```python
from build123d import *

# Parameters (mm, degrees)
ESQUISSE1_R        = 1.5
BOSS_EXTRU_2_DEPTH = 3


with BuildPart() as part:
    # Esquisse1 → Boss.-Extru.2 (new body)
    with BuildSketch(Plane.XY):
        with BuildLine():
            Line((10, -16.155494421), (10, -33.155494421))
            Line((10, -33.155494421), (-10, -33.155494421))
            Line((-10, -33.155494421), (-10, -16.155494421))
            ThreePointArc((-10, -16.155494421), (0, 19), (10, -16.155494421))
        make_face()
        with Locations((0, 14)):
            Circle(ESQUISSE1_R, mode=Mode.SUBTRACT)
        with Locations((12.124355653, -7)):
            Circle(ESQUISSE1_R, mode=Mode.SUBTRACT)
        with Locations((-12.124355653, -7)):
            Circle(ESQUISSE1_R, mode=Mode.SUBTRACT)
        with BuildLine():
            ThreePointArc((-2.411034891, 11.820685714), (0, 10.75), (2.411034891, 11.820685714))
            ThreePointArc((2.411034891, 11.820685714), (3.975330286, 12.779130538), (5.80943088, 12.737759334))
            ThreePointArc((5.80943088, 12.737759334), (11.865562564, 7.430237213), (13.995977593, -0.335575935))
            ThreePointArc((13.995977593, -0.335575935), (13.382779595, -2.564868949), (11.442531564, -3.822325392))
            ThreePointArc((11.442531564, -3.822325392), (9.309773091, -5.375), (9.031496673, -7.998360322))
            ThreePointArc((9.031496673, -7.998360322), (9.079386541, -9.832302285), (8.126507731, -11.399994391))
            ThreePointArc((8.126507731, -11.399994391), (0.5019929, -13.990997217), (-7.288606081, -11.953084179))
            ThreePointArc((-7.288606081, -11.953084179), (-8.912631465, -10.307392628), (-9.031496673, -7.998360322))
            ThreePointArc((-9.031496673, -7.998360322), (-9.309773091, -5.375), (-11.442531564, -3.822325392))
            ThreePointArc((-11.442531564, -3.822325392), (-13.054716827, -2.946828253), (-13.935938611, -1.337764944))
            ThreePointArc((-13.935938611, -1.337764944), (-12.367555464, 6.560760004), (-6.707371512, 12.288660114))
            ThreePointArc((-6.707371512, 12.288660114), (-4.47014813, 12.872261577), (-2.411034891, 11.820685714))
        make_face(mode=Mode.SUBTRACT)
    extrude(amount=BOSS_EXTRU_2_DEPTH)


solid = part.part
```
Model file for the job. Use its own axes, mm. A direction names the side the tool comes from. Coordinates: 2 decimals unless noted, no trailing zeros. Write each loop counter-clockwise with the first axis right and the second up, starting at its lowest first coordinate (ties: lowest second). Pieces come first, ordered by that corner, then holes. Notation, with made-up numbers: (31.25, 89.25) - (81.25, 89.25) arc R12 cw to (81.25, 108.25) - close; hole circle Ø10 at (9.5, -3.5). An arc over 180 degrees is marked (long way). Use a Markdown table: item, result. Add a question column.
Item 1: Band-saw the part on C-C, the plane z = 1.15. Write the cut outline in (x, y).
Item 2: Band-saw the part on A-A, the plane y = -9.5. Write the cut outline in (x, z), and give its area (3 significant figures).
Item 3: 3-axis set-ups, long thin cutter, end or side, ignore diameter. For faces 1 (the face through (0, -18, 0)), 2 (the face through (10, -25, 1)), 3 (the face through (-12.4, 6.5, 1.5)): which of +Z, -Z, +X, -X, +Y, -Y reach the whole face in a straight line?
Item 4: Drop flat-ended pins along their axis: pin 1 (5 mm diameter, centred on x = 0, y = 14, fed in from -Z); pin 2 (1.5 mm diameter, centred on y = -7.5, z = 1.5, fed in from -X); pin 3 (0.9 mm diameter, centred on y = -26.5, z = 2, fed in from +X); pin 4 (1 mm diameter, centred on x = -10, z = 0.5, fed in from +Y). Give the stop position or say it passes through.
Item 5: Drill centre lines: line 1 along Y through (x, z) = (-12, 0.7); line 2 along Y through (x, z) = (11, 0.6); line 3 along Y through (x, z) = (2.5, 2.8). Where is each one in solid material? Low to high.
Item 6: Two-plate mould, pull along X, no slides. Class faces 4 (the face through (-10, -25, 1)), 5 (the face through (0, -33.155, 1)), 6 (the face through (0.616, -13.986, 1.479)), 7 (the face through (-11.43, -8.33, 1.48)): pulls with the +X half, pulls with the -X half, needs draft (parallel to the pull), parting line crosses it, or undercut.
Item 7: Band-saw the part on B-B, the plane x = 0. Write the cut outline in (y, z), and give its area (3 significant figures).
Item 8: Band-saw the part on D-D, the plane y = -18.5. Write the cut outline in (x, z).
A:
| question | item | result |
|---|---|---|
| 1 | outline | (-10, -33.16) - (10, -33.16) - (10, -16.16) arc R19 ccw (long way) to (-10, -16.16) - close; hole (-13.94, -1.34) arc R3.25 ccw to (-11.44, -3.82) arc R3.25 cw to (-9.03, -8) arc R3.25 ccw to (-7.29, -11.95) arc R14 ccw to (8.13, -11.4) arc R3.25 ccw to (9.03, -8) arc R3.25 cw to (11.44, -3.82) arc R3.25 ccw to (14, -0.34) arc R14 ccw to (5.81, 12.74) arc R3.25 ccw to (2.41, 11.82) arc R3.25 cw to (-2.41, 11.82) arc R3.25 ccw to (-6.71, 12.29) arc R14 ccw to start; hole circle Ø3 at (-12.12, -7); hole circle Ø3 at (0, 14); hole circle Ø3 at (12.12, -7) |
| 2 | outline | (-16.45, 0) - (-9.15, 0) - (-9.15, 3) - (-16.45, 3) - close; (9.15, 0) - (16.45, 0) - (16.45, 3) - (9.15, 3) - close |
| 2 | area | 43.8 mm² |
| 3 | face 1 | -Z, +X, -X, +Y, -Y |
| 3 | face 2 | +Z, -Z, +X, -Y |
| 3 | face 3 | +Z, -Z |
| 4 | pin 1 | stops at z = 0 |
| 4 | pin 2 | stops at x = -17.76 |
| 4 | pin 3 | stops at x = 10 |
| 4 | pin 4 | stops at y = 16.45 |
| 5 | line 1 | y = -14.73 to -8.49, -5.51 to -3.65, 7.21 to 14.73 |
| 5 | line 2 | y = -15.49 to -7.99, -6.01 to -3.95, 8.66 to 15.49 |
| 5 | line 3 | y = -33.16 to -13.77, 11.92 to 18.83 |
| 6 | face 4 | pulls with the -X half |
| 6 | face 5 | needs draft |
| 6 | face 6 | undercut |
| 6 | face 7 | undercut |
| 7 | outline | (-33.16, 0) - (-14, 0) - (-14, 3) - (-33.16, 3) - close; (10.75, 0) - (12.5, 0) - (12.5, 3) - (10.75, 3) - close; (15.5, 0) - (19, 0) - (19, 3) - (15.5, 3) - close |
| 7 | area | 73.2 mm² |
| 8 | outline | (-10, 0) - (10, 0) - (10, 3) - (-10, 3) - close |
